from build123d import *

# Parameters (mm, degrees)
BOSS_EXTRUDE1_DEPTH = 7.5
CHAMFER1_SIZE       = 2.5
SKETCH2_R           = 5
BOSS_EXTRUDE2_DEPTH = 10
SKETCH3_R           = 5
CUT_EXTRUDE1_DEPTH  = 10


with BuildPart() as part:
    # Sketch1 → Boss-Extrude1 (new, symmetric)
    with BuildSketch(Plane.YZ):
        with BuildLine():
            ThreePointArc((-82.746539792, 19.872642429), (-104.801791361, 2.808746854), (-88.361833105, -19.715427415))
            ThreePointArc((-88.361833105, -19.715427415), (0.256800738, -25.931146508), (88.369675456, -14.61660998))
            ThreePointArc((88.369675456, -14.61660998), (99.852333231, 2.099570811), (84.186105477, 14.977902914))
            ThreePointArc((84.186105477, 14.977902914), (0.617423728, 13.934366249), (-82.746539792, 19.872642429))
        make_face()
    extrude(amount=BOSS_EXTRUDE1_DEPTH, both=True)

    # Chamfer1
    chamfer1_edges = [part.edges().sort_by_distance(p)[0] for p in [
        (7.5, 0.256800738, -25.931146508),
        (7.5, 99.852333231, 2.099570811),
        (7.5, 0.617423728, 13.934366249),
        (-7.5, 99.852333231, 2.099570811),
        (-7.5, 0.256800738, -25.931146508),
        (-7.5, -104.801791361, 2.808746854),
        (-7.5, 0.617423728, 13.934366249),
        (7.5, -104.801791361, 2.808746854),
    ]]
    chamfer(chamfer1_edges, length=CHAMFER1_SIZE)

    # Sketch2 → Boss-Extrude2 (add)
    with BuildSketch(Plane(origin=(-7.5, 0, 0), x_dir=(0, -1, 0), z_dir=(-1, 0, 0))):
        with Locations(Location((85, 0, 0), (0, 0, 270))):
            Circle(SKETCH2_R)
    extrude(amount=BOSS_EXTRUDE2_DEPTH)

    # Sketch3 → Cut-Extrude1 (cut)
    with BuildSketch(Plane.YZ.offset(7.5)):
        with Locations(Location((85, 0, 0), (0, 0, 270))):
            Circle(SKETCH3_R)
    extrude(amount=-CUT_EXTRUDE1_DEPTH, mode=Mode.SUBTRACT)


solid = part.part
Work out the finished part from the listing and answer in its coordinate system (mm). A direction names the side the tool comes from. Round coordinates to 2 decimals unless told otherwise and drop trailing zeros. Loops run counter-clockwise (first coordinate to the right, second up) from the corner with the lowest first, then second, coordinate; pieces in that order, holes last. Notation, with made-up numbers: (-32, 17) -> (-22, 17) arc R17 ccw to (-22, 48) -> close; hole circle Ø9 at (78.25, -22.5). An arc over 180 degrees is marked (long way). Use one line per item in the form item = value.
(1) Find section C-C on x = -13.25. Give the vertices of the cut face in (y, z).
Answer list:
outline = circle Ø10 at (-85, 0)
(2) Find section A-A on z = 0. Give the vertices of the cut face in (x, y), then the cut area to 3 significant figures.
Answer list:
outline = (-17.5, -90) -> (-7.5, -90) -> (-7.5, -102.5) -> (-5, -105) -> (5, -105) -> (7.5, -102.5) -> (7.5, 80) -> (-2.5, 80) -> (-2.5, 90) -> (7.5, 90) -> (7.5, 97.5) -> (5, 100) -> (-5, 100) -> (-7.5, 97.5) -> (-7.5, -80) -> (-17.5, -80) -> close
area = 3,060 mm2
(3) Find section B-B on x = 3. Give the vertices of the cut face in (y, z).
Answer list:
outline = (-88.36, -19.72) arc R450 ccw to (88.37, -14.62) arc R15 ccw to (84.19, 14.98) arc R1000 cw to (-82.75, 19.87) arc R20 ccw to start; hole circle Ø10 at (85, 0)
(4) For a pull along Y with two mould halves and no side action, classify faces 3 (the flat face through (-17.5, -85, 0)), 4 (the cylindrical face through (-12.43, -80.12, 1.08)), 5 (the flat face through (-2.5, 85, 0)) as released by +Y, released by -Y, zero draft, split by the parting line, or undercut.
Answer list:
face_3 = zero draft
face_4 = split by the parting line
face_5 = undercut
(5) Flat-ended cylindrical pins translate along their axes: P1, Ø9, axis at y = 85, z = 0, coming from the -X side; P2, Ø1, axis at x = -2.5, z = 11.5, coming from the -Y side; P3, Ø3, axis at y = 84.5, z = -0.5, coming from the +X side. Find the tip coordinate at first contact, or state that the pin passes through.
Answer list:
P1 = -7.5
P2 = -101.7
P3 = -2.5
(6) Straight lines are drawn through the part: line 1 (Y direction, x = 1.25, z = 0); line 2 (X direction, y = -97, z = 4.5); line 3 (Y direction, x = -0.5, z = -2.5). For each, find the intervals that lie inside material, in ascending order.
Answer list:
line_1 = -105 to 80, 90 to 100
line_2 = -7.5 to 7.5
line_3 = -104.84 to 80.67, 89.33 to 99.79
(7) A tool of negligible diameter and unlimited length cuts with its end or side. For faces 1 (the flat face through (7.5, -4, -3)), 2 (the cylindrical face through (2.57, 80.12, 1.08)), from which of +Z, -Z, +X, -X, +Y, -Y can it reach the whole face along a straight path? Write none if from no direction.
Answer list:
face_1 = +Z, -Z, +X, +Y, -Y
face_2 = +X
